from build123d import *

# Parameters (mm, degrees)
F0_R     = 40.6727472004
F0_R_2   = 11.7636370253
F1_DEPTH = 12.7
F2_R     = 12.69999
F3_DEPTH = 50.8


# Not quite as in the source:
# - a fillet or chamfer is up to 0.001 mm smaller than in the source, because OpenCascade refuses the exact size
# - the program builds the solid bodies; features that only make, move or delete a surface that nothing else refers to are left out


with BuildPart() as f1:
    # F0 (on Top) → F1 (new body)
    with BuildSketch(Plane.XY):
        Circle(F0_R)
        Circle(F0_R_2, mode=Mode.SUBTRACT)
    extrude(amount=F1_DEPTH)

    # F2 (radius 12.7 in the source; OpenCascade refuses exactly that, so slightly less here)
    f2_edges = [f1.edges().sort_by_distance(p)[0] for p in [
        (-40.672747, 0, 12.7),
    ]]
    fillet(f2_edges, radius=F2_R)

    # F0 (on Top) → F3 (join)
    with BuildSketch(Plane.XY):
        Circle(F0_R_2)
    extrude(amount=F3_DEPTH)


solid = f1.part
Here's how the part is built. I have some questions about the finished solid (model axes, mm). A direction names the side the tool comes from. Round coordinates to 2 decimals unless told otherwise and drop trailing zeros. Loops run counter-clockwise (first coordinate to the right, second up) from the corner with the lowest first, then second, coordinate; pieces in that order, holes last.
1. If we section it at C-C on z = 43: Write out the boundary of the cut face in (x, y), plus the area to 3 significant figures.
Answer list:
outline: circle Ø23.53 at (0, 0)
area: 435 mm2
2. For P1, Ø8, axis at x = -27.5, y = -7, coming from the +Z side; P2, Ø1, axis at x = -15.5, y = -28, coming from the -Z side; P3, Ø2, axis at y = -11.5, z = 26.5, coming from the +X side, each with a flat end and sliding along its axis, tell me the tip position at first contact or that it passes through.
Answer list:
P1: stops at z = 12.7
P2: stops at z = 0
P3: stops at x = 5.3
3. If I drill on line 1 along X through (y, z) = (0.5, 20.5); line 2 along Z through (x, y) = (-18.5, -1); line 3 along Y through (x, z) = (14, 4), over which ranges is the centre line in solid material (lowest first)?
Answer list:
line 1: x = -11.75 to 11.75
line 2: z = 0 to 12.7
line 3: y = -37.5 to 37.5
4. Which directions (+Z, -Z, +X, -X, +Y, -Y) give clear straight access to the entire face, cutting with the end or side of a thin tool? Please do faces 1 (the face through (-2.55, -11.484, 31.483)), 2 (the face through (0, 0, 50.8)).
Answer list:
face 1: +Z
face 2: +Z, +X, -X, +Y, -Y
